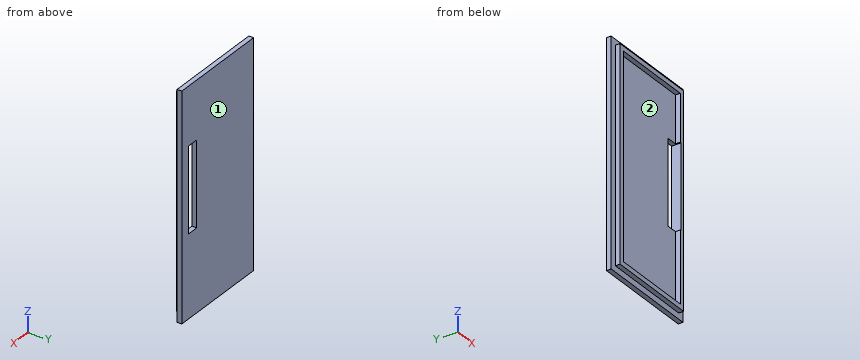
Autodesk Inventor part; units mm, degrees
ref_plane "YZ Plane" through (0, 0, 0) normal (1, 0, 0) x (0, 1, 0)
ref_plane "XZ Plane" through (0, 0, 0) normal (0, 1, 0) x (-1, 0, 0)
ref_plane "XY Plane" through (0, 0, 0) normal (0, 0, 1) x (1, 0, 0)
sketch "Sketch1" plane through (0, 0, 0) normal (0, 1, 0) x (-1, 0, 0)
  line L0 (20.49, -1.25) -> (1.25, -1.25)
  line L1 (1.25, -1.25) -> (1.25, -45.89)
  line L2 (1.25, -45.89) -> (20.49, -45.89)
  line L3 (20.49, -45.89) -> (20.49, -1.25)
  line L4 (18.49, -3.25) -> (3.25, -3.25) construction
  line L5 (3.25, -3.25) -> (3.25, -43.89) construction
  line L6 (3.25, -43.89) -> (18.49, -43.89) construction
  line L7 (18.49, -43.89) -> (18.49, -3.25) construction
  circle A0 centre (18.49, -3.25) radius 2 construction
  circle A1 centre (18.49, -3.25) radius 0.75 construction
  circle A2 centre (18.49, -43.89) radius 2 construction
  circle A3 centre (18.49, -43.89) radius 0.75 construction
  circle A4 centre (3.25, -43.89) radius 2 construction
  circle A5 centre (3.25, -43.89) radius 0.75 construction
  circle A6 centre (3.25, -3.25) radius 2 construction
  circle A7 centre (3.25, -3.25) radius 0.75 construction
  line L8 (0, -47.14) -> (21.74, -47.14)
  line L9 (21.74, -47.14) -> (21.74, 0)
  line L10 (21.74, 0) -> (0, 0)
  line L11 (0, 0) -> (0, -47.14)
  line L12 (19.49, -2.25) -> (2.25, -2.25)
  line L13 (2.25, -2.25) -> (2.25, -44.89)
  line L14 (2.25, -44.89) -> (19.49, -44.89)
  line L15 (19.49, -44.89) -> (19.49, -2.25)
  dimension "d2" = 40.64
  dimension "d3" = 15.24
  dimension "d4" = 1.5
  dimension "d5" = 4
  dimension "d6" = 1.25
  dimension "d7" = 1.25
  dimension "d8" = 1.25
  dimension "d9" = 1.25
  dimension "d12" = 1
  dimension "d13" = 1
  dimension "d14" = 1
  dimension "d15" = 1
extrude "Extrusion1" add sketch "Sketch1" against normal blind 1 contours L3 L2 L1 L0
extrude "Extrusion2" add sketch "Sketch1" along normal blind 1 contours L3 L2 L1 L0 | L11 L10 L9 L8 | L15 L14 L13 L12
sketch "Sketch2" plane through (0, -1, 0) normal (0, -1, 0) x (1, 0, 0)
  line L0 (-4.52, -29.92) -> (-1.98, -29.92)
  line L1 (-1.98, -29.92) -> (-1.98, -12.14)
  line L2 (-1.98, -12.14) -> (-4.52, -12.14)
  line L3 (-4.52, -12.14) -> (-4.52, -29.92)
  circle A0 centre (-3.25, -28.65) radius 0.508 construction
  circle A1 centre (-3.25, -13.41) radius 0.508 construction
  point P0 (0, 0)
  point P1 (-3.25, -29.92)
  dimension "d20" = 2.54
  dimension "d21" = 17.78
  dimension "d22" = 15.24
  dimension "d23" = 1.27
  dimension "d24" = 1.27
extrude "Extrusion3" cut sketch "Sketch2" against normal through all
equation "\"d7\" = d6"
equation "\"d8\" = d7"
equation "\"d9\" = d7"
equation "\"d21\" = 7 * d20"
equation "\"d24\" = 0.5 * d20"
properties part number "Arduino Lid"
Source: CAD feature listing. Evaluate the final solid. Frame: model axes, mm. Face numbers are marked on the shaded views. Coordinates: 2 decimals unless noted, no trailing zeros. Write each loop counter-clockwise with the first axis right and the second up, starting at its lowest first coordinate (ties: lowest second). Pieces come first, ordered by that corner, then holes. Notation, with made-up numbers: (-38, 42.25) -> (-19, 42.25) arc R30 cw to (-19, 70.25) -> close; hole circle Ø11 at (-31, -19.5). An arc over 180 degrees is marked (long way). Return JSON: item names as keys, results as strings. Group by question number.
1) Section query A-A, the plane z = -27. Return loops of the section in (x, y).
2) Section query C-C, the plane y = -0.5. Return loops of the section in (x, z).
3) Section query D-D, the plane x = -15.5. Return loops of the section in (y, z).
4) Contact query for flat-ended pins moving along their axis: P1, Ø1.5, axis at x = -3.5, z = -14, coming from the -Y side; P2, Ø0.8, axis at x = -14, y = -0.5, coming from the +Z side; P3, Ø5, axis at x = -10, z = -13, coming from the -Y side; P4, Ø0.5, axis at y = -0.5, z = -21.5, coming from the +X side. Output: stop coordinate, or through.
5) Ray query, line 1 along X through (y, z) = (-0.8, -26.5); line 2 along Z through (x, y) = (-12.5, -0.75); line 3 along X through (y, z) = (-0.05, -3.5). Return the intervals inside material, ascending.
6) Section query B-B, the plane x = -3.25. Return loops of the section in (y, z), plus the area to 3 significant figures.
7) Mould query, pull axis Z, two halves, no side actions, for the marked faces 1 and 2. Classes: +Z half, -Z half, draft (parallel to the pull), parting line (faces both ways), or undercut.
From the geometry:
{
 "1": {"outline": "(-21.74, 0) -> (-20.49, 0) -> (-20.49, -1) -> (-19.49, -1) -> (-19.49, 0) -> (-4.52, 0) -> (-4.52, 1) -> (-21.74, 1) -> close; (-1.98, -1) -> (-1.25, -1) -> (-1.25, 0) -> (0, 0) -> (0, 1) -> (-1.98, 1) -> close"},
 "2": {"outline": "(-20.49, -45.89) -> (-1.25, -45.89) -> (-1.25, -1.25) -> (-20.49, -1.25) -> close; hole (-19.49, -44.89) -> (-2.25, -44.89) -> (-2.25, -29.92) -> (-1.98, -29.92) -> (-1.98, -12.14) -> (-2.25, -12.14) -> (-2.25, -2.25) -> (-19.49, -2.25) -> close"},
 "3": {"outline": "(-1, -45.89) -> (0, -45.89) -> (0, -47.14) -> (1, -47.14) -> (1, 0) -> (0, 0) -> (0, -1.25) -> (-1, -1.25) -> (-1, -2.25) -> (0, -2.25) -> (0, -44.89) -> (-1, -44.89) -> close"},
 "4": {"P1": "through", "P2": "z = -1.25", "P3": "y = 0", "P4": "x = -1.25"},
 "5": {"line 1": "-20.49 to -19.49, -1.98 to -1.25", "line 2": "-45.89 to -44.89, -2.25 to -1.25", "line 3": "-20.49 to -19.49, -2.25 to -1.25"},
 "6": {"outline": "(-1, -45.89) -> (0, -45.89) -> (0, -47.14) -> (1, -47.14) -> (1, -29.92) -> (0, -29.92) -> (0, -44.89) -> (-1, -44.89) -> close; (-1, -2.25) -> (0, -2.25) -> (0, -12.14) -> (1, -12.14) -> (1, 0) -> (0, 0) -> (0, -1.25) -> (-1, -1.25) -> close", "area": "31.4 mm²"},
 "7": {"face 1": "draft", "face 2": "undercut"}
}
